```python
from build123d import *

# Parameters (mm, degrees)
EXTRUDE_DEPTH = 20
FILLET_R      = 1.5


with BuildPart() as part:
    # Sketch → Extrude (new body)
    with BuildSketch(Plane.XY):
        Polygon((31, 0), (31, 5), (6, 5), (6, 47), (7.5, 47), (7.5, 55), (27.5, 55), (27.5, 47), (32.5, 47), (32.5, 55), (32.5, 60), (6, 60), (0, 60), (0, 0), (6, 0), align=None)
    extrude(amount=EXTRUDE_DEPTH)

    # Fillet
    fillet_edges = [part.edges().sort_by_distance(p)[0] for p in [
        (0, 60, 10),
        (0, 0, 10),
        (31, 0, 10),
        (31, 5, 10),
        (27.5, 47, 10),
        (32.5, 47, 10),
        (32.5, 60, 10),
    ]]
    fillet(fillet_edges, radius=FILLET_R)


solid = part.part
```
Build history of the part. All positions in model axes, mm. A direction names the side the tool comes from. Coordinates: 2 decimals unless noted, no trailing zeros. Order: outer loops, then holes, each group sorted by start corner. A loop starts at its lowest first (then second) coordinate and runs counter-clockwise, first axis right, second up.
Item 1: Drill centre lines: L1, parallel to Y at x = 29.5, z = 17; L2, parallel to Y at x = 23.5, z = 15.5; L3, parallel to X at y = 52.5, z = 17.25. Where is each one in solid material? Low to high.
Filled in:
L1: y = 0 to 5, 47 to 60
L2: y = 0 to 5, 55 to 60
L3: x = 0 to 7.5, 27.5 to 32.5
Item 2: Drop flat-ended pins along their axis: pin 1 Ø6 at (y, z) = (19.5, 6) entering from +X; pin 2 Ø2 at (y, z) = (2.5, 12) entering from +X; pin 3 Ø12 at (x, y) = (7, 8) entering from -Z; pin 4 Ø12 at (x, y) = (15.5, 27.5) entering from -Z. Give the stop position or say it passes through.
Filled in:
pin 1: stops at x = 6
pin 2: stops at x = 31
pin 3: stops at z = 0
pin 4: passes through
Item 3: Tool access for faces 1 (the flat face through (6, 26, 10)), 2 (the flat face through (7.5, 51, 10)), 3 (the flat face through (31, 2, 10)): list every direction of +Z, -Z, +X, -X, +Y, -Y with a clear straight run to the whole face (end or side of a thin tool).
Filled in:
face 1: +Z, -Z, +X
face 2: +Z, -Z
face 3: +Z, -Z, +X, -Y
Item 4: Saw through at D-D on y = 17. List the corners of the cut face in (x, z).
Filled in:
outline: (0, 0) - (6, 0) - (6, 20) - (0, 20) - close
Item 5: Saw through at A-A on y = 53. List the corners of the cut face in (x, z), then the cut area to 3 significant figures.
Filled in:
outline: (0, 0) - (7.5, 0) - (7.5, 20) - (0, 20) - close; (27.5, 0) - (32.5, 0) - (32.5, 20) - (27.5, 20) - close
area: 250 mm2
Item 6: Saw through at B-B on x = 9.5. List the corners of the cut face in (y, z), then the cut area to 3 significant figures.
Filled in:
outline: (0, 0) - (5, 0) - (5, 20) - (0, 20) - close; (55, 0) - (60, 0) - (60, 20) - (55, 20) - close
area: 200 mm2
Item 7: Saw through at C-C on z = 6.75. List the corners of the cut face in (x, y).
Filled in:
outline: (0, 1.5) arc R1.5 ccw to (1.5, 0) - (29.5, 0) arc R1.5 ccw to (31, 1.5) - (31, 3.5) arc R1.5 ccw to (29.5, 5) - (6, 5) - (6, 47) - (7.5, 47) - (7.5, 55) - (27.5, 55) - (27.5, 48.5) arc R1.5 ccw to (29, 47) - (31, 47) arc R1.5 ccw to (32.5, 48.5) - (32.5, 58.5) arc R1.5 ccw to (31, 60) - (1.5, 60) arc R1.5 ccw to (0, 58.5) - close
Item 8: Mould opens along X. For faces 4 (the cylindrical face through (30.57, 4.55, 10.14)), 5 (the flat face through (7, 47, 10)), 6 (the flat face through (27.5, 52, 10)) say: released by +X, released by -X, zero draft, split by the parting line, or undercut.
Filled in:
face 4: released by +X
face 5: zero draft
face 6: undercut
